Model file for the job. Use its own axes, mm. A direction names the side the tool comes from. Round coordinates to 2 decimals unless told otherwise and drop trailing zeros. Loops run counter-clockwise (first coordinate to the right, second up) from the corner with the lowest first, then second, coordinate; pieces in that order, holes last. Notation, with made-up numbers: (38, 68.5) -> (96, 68.5) arc R20 cw to (96, 74.5) -> close; hole circle Ø10 at (20, 54.25). An arc over 180 degrees is marked (long way). Use a Markdown table: item, result. Add a question column.
```python
from build123d import *

# Parameters (mm, degrees)
F3_W         = 27
F3_H         = 27
F4_DEPTH     = 30
F5_T1_DEPTH  = 950
F5_T3_DEPTH  = 986
F5_T5_DEPTH  = 902
F5_T7_DEPTH  = 938
F5_T13_DEPTH = 955
F5_T17_DEPTH = 907
F5_T20_DEPTH = 960
F5_T22_DEPTH = 998
F5_T24_DEPTH = 953
F5_T26_DEPTH = 950
F5_T28_DEPTH = 905
F5_T30_DEPTH = 912
F5_T36_DEPTH = 910
F5_T40_DEPTH = 958
F5_T47_DEPTH = 910
F5_T51_DEPTH = 958
F8_D         = 5
F8_ON_F6_D   = 5


# Not quite as in the source:
# - a fillet or chamfer that OpenCascade refuses, or shapes differently, is made with other operations: its cross-section is extruded or revolved along the edge and cut away or added


with BuildPart() as f2:
    # F2: sweep along a path in F1
    with BuildLine(Plane.XY) as f2_path:
        Line((0, 0), (0, -948))
        Line((0, -948), (-900, -948))
    # F0 (on Front) → F2 (sweep)
    with BuildSketch(Plane.XZ):
        Polygon((38, -2), (38, -25), (40, -25), (40, 0), (0, 0), (0, -350), (27, -350), (27, -376), (29, -376), (29, -348), (2, -348), (2, -2), align=None)
    sweep(path=f2_path.line, transition=Transition.RIGHT)

    # F3 (on face) → F4 (cut)
    with BuildSketch(Plane.XY.offset(-348)):
        with Locations((15.5, -963.5)):
            Rectangle(F3_W, F3_H)
    extrude(amount=-F4_DEPTH, mode=Mode.SUBTRACT)

    # F5: fillet of radius 2 on 15 edges, made by hand

    # F5_s2 → F5_t1 (join)
    with BuildSketch(Plane.XZ):
        with BuildLine():
            ThreePointArc((2, -346), (2.5857864376, -347.4142135624), (4, -348))
            Line((4, -348), (2, -348))
            Line((2, -348), (2, -346))
        make_face()
        with BuildLine():
            ThreePointArc((25, -350), (26.4142135624, -350.5857864376), (27, -352))
            Line((27, -352), (27, -350))
            Line((27, -350), (25, -350))
        make_face()
        with BuildLine():
            ThreePointArc((4, -2), (2.5857864376, -2.5857864376), (2, -4))
            Line((2, -4), (2, -2))
            Line((2, -2), (4, -2))
        make_face()
    extrude(amount=F5_T1_DEPTH)

    # F5_s4 → F5_t3 (join)
    with BuildSketch(Plane.XZ):
        with BuildLine():
            ThreePointArc((38, -4), (37.4142135624, -2.5857864376), (36, -2))
            Line((36, -2), (38, -2))
            Line((38, -2), (38, -4))
        make_face()
    extrude(amount=F5_T3_DEPTH)

    # F5_s6 → F5_t5 (join)
    with BuildSketch(Plane.YZ.offset(-900)):
        with BuildLine():
            ThreePointArc((-973, -350), (-974.4142135624, -350.5857864376), (-975, -352))
            Line((-975, -352), (-975, -350))
            Line((-975, -350), (-973, -350))
        make_face()
        with BuildLine():
            ThreePointArc((-952, -2), (-950.5857864376, -2.5857864376), (-950, -4))
            Line((-950, -4), (-950, -2))
            Line((-950, -2), (-952, -2))
        make_face()
    extrude(amount=F5_T5_DEPTH)

    # F5_s8 → F5_t7 (join)
    with BuildSketch(Plane.YZ.offset(-900)):
        with BuildLine():
            ThreePointArc((-984, -2), (-985.4142135624, -2.5857864376), (-986, -4))
            Line((-986, -4), (-986, -2))
            Line((-986, -2), (-984, -2))
        make_face()
    extrude(amount=F5_T7_DEPTH)


with BuildPart() as f5_tool11:
    # F5_s12 → F5_t13 (new body)
    with BuildSketch(Plane.XZ):
        with BuildLine():
            ThreePointArc((4, -2), (2.5857864376, -2.5857864376), (2, -4))
            Line((2, -4), (2, -2))
            Line((2, -2), (4, -2))
        make_face()
    extrude(amount=F5_T13_DEPTH)

    split(bisect_by=Plane.XZ.offset(950), keep=Keep.TOP)


with BuildPart() as f5_tool15:
    # F5_s16 → F5_t17 (new body)
    with BuildSketch(Plane.YZ.offset(7)):
        with BuildLine():
            ThreePointArc((-952, -2), (-950.5857864376, -2.5857864376), (-950, -4))
            Line((-950, -4), (-950, -2))
            Line((-950, -2), (-952, -2))
        make_face()
    extrude(amount=-F5_T17_DEPTH)

    split(bisect_by=Plane.YZ.offset(2), keep=Keep.TOP)


with BuildPart() as f5_tool11_1:
    add(f5_tool11.part)

    # F5_t19: intersect F5_tool15
    add(f5_tool15.part, mode=Mode.INTERSECT)


with BuildPart() as f2_1:
    add(f2.part)

    # F5_t9: union F5_tool11
    add(f5_tool11_1.part)

    # F5_s21 → F5_t20 (cut)
    with BuildSketch(Plane.XZ.offset(-5)):
        with BuildLine():
            ThreePointArc((27, -348), (28.4142135624, -348.5857864376), (29, -350))
            Line((29, -350), (29, -348))
            Line((29, -348), (27, -348))
        make_face()
    extrude(amount=F5_T20_DEPTH, mode=Mode.SUBTRACT)

    # F5_s23 → F5_t22 (cut)
    with BuildSketch(Plane.XZ.offset(-5)):
        with BuildLine():
            ThreePointArc((38, 0), (39.4142135624, -0.5857864376), (40, -2))
            Line((40, -2), (40, 0))
            Line((40, 0), (38, 0))
        make_face()
    extrude(amount=F5_T22_DEPTH, mode=Mode.SUBTRACT)

    # F5_s25 → F5_t24 (cut)
    with BuildSketch(Plane.XZ.offset(-5)):
        with BuildLine():
            ThreePointArc((0, -2), (0.5857864376, -0.5857864376), (2, 0))
            Line((2, 0), (0, 0))
            Line((0, 0), (0, -2))
        make_face()
        with BuildLine():
            ThreePointArc((2, -350), (0.5857864376, -349.4142135624), (0, -348))
            Line((0, -348), (0, -350))
            Line((0, -350), (2, -350))
        make_face()
    extrude(amount=F5_T24_DEPTH, mode=Mode.SUBTRACT)

    # F5_s27 → F5_t26 (cut)
    with BuildSketch(Plane.YZ.offset(-905)):
        with BuildLine():
            ThreePointArc((-988, -2), (-987.4142135624, -0.5857864376), (-986, 0))
            Line((-986, 0), (-988, 0))
            Line((-988, 0), (-988, -2))
        make_face()
    extrude(amount=F5_T26_DEPTH, mode=Mode.SUBTRACT)

    # F5_s29 → F5_t28 (cut)
    with BuildSketch(Plane.YZ.offset(-905)):
        with BuildLine():
            ThreePointArc((-948, -2), (-948.5857864376, -0.5857864376), (-950, 0))
            Line((-950, 0), (-948, 0))
            Line((-948, 0), (-948, -2))
        make_face()
        with BuildLine():
            ThreePointArc((-948, -348), (-948.5857864376, -349.4142135624), (-950, -350))
            Line((-950, -350), (-948, -350))
            Line((-948, -350), (-948, -348))
        make_face()
    extrude(amount=F5_T28_DEPTH, mode=Mode.SUBTRACT)

    # F5_s31 → F5_t30 (cut)
    with BuildSketch(Plane.YZ.offset(-905)):
        with BuildLine():
            ThreePointArc((-977, -350), (-976.4142135624, -348.5857864376), (-975, -348))
            Line((-975, -348), (-977, -348))
            Line((-977, -348), (-977, -350))
        make_face()
    extrude(amount=F5_T30_DEPTH, mode=Mode.SUBTRACT)


with BuildPart() as f5_tool34:
    # F5_s35 → F5_t36 (new body)
    with BuildSketch(Plane.YZ.offset(5)):
        with BuildLine():
            ThreePointArc((-948, -2), (-948.5857864376, -0.5857864376), (-950, 0))
            Line((-950, 0), (-948, 0))
            Line((-948, 0), (-948, -2))
        make_face()
    extrude(amount=-F5_T36_DEPTH)

    split(bisect_by=Plane.YZ, keep=Keep.TOP)


with BuildPart() as f5_tool38:
    # F5_s39 → F5_t40 (new body)
    with BuildSketch(Plane.XZ.offset(-5)):
        with BuildLine():
            ThreePointArc((0, -2), (0.5857864376, -0.5857864376), (2, 0))
            Line((2, 0), (0, 0))
            Line((0, 0), (0, -2))
        make_face()
    extrude(amount=F5_T40_DEPTH)

    split(bisect_by=Plane.XZ.offset(948), keep=Keep.TOP)


with BuildPart() as f5_tool34_1:
    add(f5_tool34.part)

    # F5_t42: intersect F5_tool38
    add(f5_tool38.part, mode=Mode.INTERSECT)


with BuildPart() as f2_2:
    add(f2_1.part)

    # F5_t32: cut F5_tool34
    add(f5_tool34_1.part, mode=Mode.SUBTRACT)


with BuildPart() as f5_tool45:
    # F5_s46 → F5_t47 (new body)
    with BuildSketch(Plane.YZ.offset(5)):
        with BuildLine():
            ThreePointArc((-948, -348), (-948.5857864376, -349.4142135624), (-950, -350))
            Line((-950, -350), (-948, -350))
            Line((-948, -350), (-948, -348))
        make_face()
    extrude(amount=-F5_T47_DEPTH)

    split(bisect_by=Plane.YZ, keep=Keep.TOP)


with BuildPart() as f5_tool49:
    # F5_s50 → F5_t51 (new body)
    with BuildSketch(Plane.XZ.offset(-5)):
        with BuildLine():
            ThreePointArc((2, -350), (0.5857864376, -349.4142135624), (0, -348))
            Line((0, -348), (0, -350))
            Line((0, -350), (2, -350))
        make_face()
    extrude(amount=F5_T51_DEPTH)

    split(bisect_by=Plane.XZ.offset(948), keep=Keep.TOP)


with BuildPart() as f5_tool45_1:
    add(f5_tool45.part)

    # F5_t53: intersect F5_tool49
    add(f5_tool49.part, mode=Mode.INTERSECT)


with BuildPart() as f2_3:
    add(f2_2.part)

    # F5_t43: cut F5_tool45
    add(f5_tool45_1.part, mode=Mode.SUBTRACT)

    # F8 (through all)
    with Locations(Plane(origin=(0, -975, 0), x_dir=(-1, 0, 0), z_dir=(0, 1, 0))):
        with Locations((98, -364), (449, -364), (800, -364)):
            Hole(F8_D / 2)

    # F8 on F6 (through all)
    with Locations(Plane(origin=(27, 0, 0), x_dir=(0, -1, 0), z_dir=(-1, 0, 0))):
        with Locations((100, -364), (475, -364), (850, -364)):
            Hole(F8_ON_F6_D / 2)


solid = f2_3.part
```
1) Cut at A-A on x = -681. Write the cut outline in (y, z).
2) Wall check: probe 1 along Z at (x, y) = (27.95, -475); probe 2 along X at (y, z) = (-976, -364); probe 3 along Y at (x, z) = (28.65, -364). Give the ranges that are in metal, low to high. Write a range as from..to.
3) Cut at C-C on y = -458. Write the cut outline in (x, z), and give its area (3 significant figures).
4) Pin check, flat tips, straight feed: pin 1 Ø2 at (x, z) = (-220.5, -150.5) entering from +Y; pin 2 Ø2 at (x, z) = (-694, -191) entering from -Y; pin 3 Ø6 at (x, z) = (-800, -364) entering from -Y. Stop position of each tip, or through.
5) Tool access for faces 1 (the face through (29, -482, -363)), 2 (the face through (-455, -975, -364)), 3 (the face through (2, -969, -349)): list every direction of +Z, -Z, +X, -X, +Y, -Y with a clear straight run to the whole face (end or side of a thin tool).
6) Pull direction Y, two halves, no side cores. Call faces 4 (the face through (-456, -948, -173)), 5 (the face through (16, -713, -2)), 6 (the face through (23, -714, 0)), 7 (the face through (-455, -977, -363)): +Y half, -Y half, draft (parallel to the pull), parting line (faces both ways), or undercut.
7) Cut at B-B on z = -185.5. Write the cut outline in (x, y).
Established:
| question | item | result |
|---|---|---|
| 1 | outline | (-988, -25) -> (-986, -25) -> (-986, -4) arc R2 cw to (-984, -2) -> (-952, -2) arc R2 cw to (-950, -4) -> (-950, -348) -> (-975, -348) arc R2 ccw to (-977, -350) -> (-977, -376) -> (-975, -376) -> (-975, -352) arc R2 cw to (-973, -350) -> (-950, -350) arc R2 ccw to (-948, -348) -> (-948, -2) arc R2 ccw to (-950, 0) -> (-986, 0) arc R2 ccw to (-988, -2) -> close |
| 2 | probe 1 | z = -376..-366.5, -361.5..-348.24, -2..0 |
| 2 | probe 2 | x = -900..-802.5, -797.5..-451.5, -446.5..-100.5, -95.5..2 |
| 2 | probe 3 | y = -950..-852.5, -847.5..-477.5, -472.5..-102.5, -97.5..0 |
| 3 | outline | (0, -348) arc R2 ccw to (2, -350) -> (25, -350) arc R2 cw to (27, -352) -> (27, -376) -> (29, -376) -> (29, -350) arc R2 ccw to (27, -348) -> (4, -348) arc R2 cw to (2, -346) -> (2, -4) arc R2 cw to (4, -2) -> (36, -2) arc R2 cw to (38, -4) -> (38, -25) -> (40, -25) -> (40, -2) arc R2 ccw to (38, 0) -> (2, 0) arc R2 ccw to (0, -2) -> close |
| 3 | area | 928 mm^2 |
| 4 | pin 1 | stops at y = -948 |
| 4 | pin 2 | stops at y = -950 |
| 4 | pin 3 | stops at y = -977 |
| 5 | face 1 | -Z, +X, +Y, -Y |
| 5 | face 2 | -Z, +X, -X, +Y |
| 5 | face 3 | -Z, +X, -Y |
| 6 | face 4 | +Y half |
| 6 | face 5 | undercut |
| 6 | face 6 | draft |
| 6 | face 7 | -Y half |
| 7 | outline | (-900, -950) -> (2, -950) -> (2, 0) -> (0, 0) -> (0, -948) -> (-900, -948) -> close |
